from build123d import *

# Parameters (mm, degrees)
BOSS_EXTRUDE1_DEPTH      = 25
BOSS_EXTRUDE2_DEPTH      = 5
BOSS_EXTRUDE2_DEPTH_BACK = 40
SKETCH6_R                = 2
CUT_EXTRUDE2_DEPTH       = 56.302200077
SKETCH7_R                = 11.5
CUT_EXTRUDE3_DEPTH       = 59.434436194
CHAMFER3_SIZE            = 2
CHAMFER4_SIZE            = 8.660254038
CHAMFER4_SIZE_2          = 5
CUT_EXTRUDE4_DEPTH       = 0.5
CUT_EXTRUDE5_DEPTH       = 0.5


with BuildPart() as part:
    # Sketch1 → Boss-Extrude1 (new, symmetric)
    with BuildSketch(Plane.XY):
        Polygon((10.103629711, 17.5), (-10.103629711, 17.5), (-20.207259422, 0), (-10.103629711, -17.5), (10.103629711, -17.5), (20.207259422, 0), align=None)
    extrude(amount=BOSS_EXTRUDE1_DEPTH, both=True)

    # Sketch2 → Boss-Extrude2 (add, two sides: drawn at the far end of the back side and taken through both)
    with BuildSketch(Plane(origin=(0, 17.5, 0), x_dir=(1, 0, 0), z_dir=(0, 1, 0)).offset(-BOSS_EXTRUDE2_DEPTH_BACK)):
        with BuildLine():
            Line((-4.788486146, -5.353793539), (-4.788486146, 5.353793539))
            ThreePointArc((-4.788486146, 5.353793539), (0, 10.142279685), (4.788486146, 5.353793539))
            Line((4.788486146, 5.353793539), (4.788486146, -5.353793539))
            ThreePointArc((4.788486146, -5.353793539), (0, -10.142279685), (-4.788486146, -5.353793539))
        make_face()
    extrude(amount=BOSS_EXTRUDE2_DEPTH + BOSS_EXTRUDE2_DEPTH_BACK)

    # Sketch6 → Cut-Extrude2 (cut, through all)
    with BuildSketch(Plane(origin=(0, 22.5, 0), x_dir=(1, 0, 0), z_dir=(0, 1, 0))):
        with Locations(Location((0, -2.5, 0), (0, 0, 270))):
            Circle(SKETCH6_R)
        with Locations(Location((0, 2.5, 0), (0, 0, 270))):
            Circle(SKETCH6_R)
    extrude(amount=-CUT_EXTRUDE2_DEPTH, mode=Mode.SUBTRACT)

    # Sketch7 → Cut-Extrude3 (cut, through all)
    with BuildSketch(Plane(origin=(0, 0, -25), x_dir=(-1, 0, 0), z_dir=(0, 0, -1))):
        Circle(SKETCH7_R)
    extrude(amount=-CUT_EXTRUDE3_DEPTH, mode=Mode.SUBTRACT)

    # Chamfer3
    chamfer3_edges = [part.edges().sort_by_distance(p)[0] for p in [
        (-15.155444566, 8.75, 25),
        (-15.155444566, -8.75, 25),
        (0, -17.5, 25),
        (15.155444566, -8.75, 25),
        (15.155444566, 8.75, 25),
        (11.5, 0, 25),
        (11.5, 0, -25),
        (15.155444566, -8.75, -25),
        (0, -17.5, -25),
        (-15.155444566, -8.75, -25),
        (0, 17.5, 25),
        (-15.155444566, 8.75, -25),
        (0, 17.5, -25),
        (15.155444566, 8.75, -25),
    ]]
    chamfer(chamfer3_edges, length=CHAMFER3_SIZE)

    # Chamfer4
    # the kernel refuses this chamfer: 8.660254038, 5 mm, written as the material it adds along each edge
    with BuildSketch(Plane(origin=(4.788486146, -17.5, -5.353793539), x_dir=(0.9998132206222078, 0.019326765612700893, 0), z_dir=(0, 0, 1))) as chamfer4_piece_1_section:
        Polygon((CHAMFER4_SIZE * 0.999813220604, -CHAMFER4_SIZE * 0.0193267656124), (-CHAMFER4_SIZE_2 * 0.0193267656127, -CHAMFER4_SIZE_2 * 0.999813220622), (0, 0), align=None)
    chamfer4_piece_1 = extrude(amount=10.707587077, mode=Mode.PRIVATE)
    chamfer4_piece_1 = split(chamfer4_piece_1, bisect_by=Plane(origin=(8.460633685, -20.345752593, 0), z_dir=(-0.8660254037844387, 0.4999999999999999, 0)), keep=Keep.TOP, mode=Mode.PRIVATE)
    chamfer4_piece_1 = split(chamfer4_piece_1, bisect_by=Plane(origin=(6.722843937, -22.5, 0), z_dir=(0, 1, 0)), keep=Keep.TOP, mode=Mode.PRIVATE)
    add(chamfer4_piece_1)
    with BuildSketch(Plane(origin=(0, -17.5, -5.353793539), x_dir=(-1, 0, 0), z_dir=(0, 0, 1))) as chamfer4_piece_2_section:
        Polygon((4.788486146 + CHAMFER4_SIZE, 0), (4.788486146, CHAMFER4_SIZE_2), (4.788486146, 0), align=None)
    chamfer4_piece_2 = revolve(axis=Axis((0, -17.5, -5.353793539), (0, -1, 0)), revolution_arc=180, mode=Mode.PRIVATE)
    chamfer4_piece_2 = split(chamfer4_piece_2, bisect_by=Plane(origin=(6.935994124, -22.986505777, -10.917233829), z_dir=(-0.8660254037844387, 0.4999999999999999, 0)), keep=Keep.TOP, mode=Mode.PRIVATE)
    chamfer4_piece_2 = split(chamfer4_piece_2, bisect_by=Plane(origin=(-6.935994098, -22.986505822, -10.917233829), z_dir=(0.8660254037844385, 0.5000000000000003, 0)), keep=Keep.TOP, mode=Mode.PRIVATE)
    chamfer4_piece_2 = split(chamfer4_piece_2, bisect_by=Plane(origin=(5.2e-08, -22.5, -10.917233829), z_dir=(0, 1, 0)), keep=Keep.TOP, mode=Mode.PRIVATE)
    add(chamfer4_piece_2)
    with BuildSketch(Plane(origin=(0, -17.5, 5.353793539), x_dir=(1, 0, 0), z_dir=(0, 0, -1))) as chamfer4_piece_3_section:
        Polygon((4.788486146 + CHAMFER4_SIZE, 0), (4.788486146, CHAMFER4_SIZE_2), (4.788486146, 0), align=None)
    chamfer4_piece_3 = revolve(axis=Axis((0, -17.5, 5.353793539), (0, -1, 0)), revolution_arc=180, mode=Mode.PRIVATE)
    chamfer4_piece_3 = split(chamfer4_piece_3, bisect_by=Plane(origin=(6.935994128, -22.98650577, 10.917233836), z_dir=(-0.8660254037844387, 0.4999999999999999, 0)), keep=Keep.TOP, mode=Mode.PRIVATE)
    chamfer4_piece_3 = split(chamfer4_piece_3, bisect_by=Plane(origin=(-6.935994097, -22.986505824, 10.917233836), z_dir=(0.8660254037844385, 0.5000000000000003, 0)), keep=Keep.TOP, mode=Mode.PRIVATE)
    chamfer4_piece_3 = split(chamfer4_piece_3, bisect_by=Plane(origin=(6.2e-08, -22.5, 10.917233836), z_dir=(0, 1, 0)), keep=Keep.TOP, mode=Mode.PRIVATE)
    add(chamfer4_piece_3)
    with BuildSketch(Plane(origin=(-4.788486146, -17.5, 5.353793539), x_dir=(-0.999813220622208, 0.019326765612700497, 0), z_dir=(0, 0, -1))) as chamfer4_piece_4_section:
        Polygon((CHAMFER4_SIZE * 0.999813220604, -CHAMFER4_SIZE * 0.0193267656124), (-CHAMFER4_SIZE_2 * 0.0193267656127, -CHAMFER4_SIZE_2 * 0.999813220622), (0, 0), align=None)
    chamfer4_piece_4 = extrude(amount=10.707587077, mode=Mode.PRIVATE)
    chamfer4_piece_4 = split(chamfer4_piece_4, bisect_by=Plane(origin=(-8.460633685, -20.345752593, 0), z_dir=(0.8660254037844385, 0.5000000000000003, 0)), keep=Keep.TOP, mode=Mode.PRIVATE)
    chamfer4_piece_4 = split(chamfer4_piece_4, bisect_by=Plane(origin=(-6.722843937, -22.5, 0), z_dir=(0, 1, 0)), keep=Keep.TOP, mode=Mode.PRIVATE)
    add(chamfer4_piece_4)
    with BuildSketch(Plane(origin=(-4.788486146, 17.5, -5.353793539), x_dir=(-0.999813220622208, -0.019326765612700497, 0), z_dir=(0, 0, 1))) as chamfer4_piece_5_section:
        Polygon((CHAMFER4_SIZE * 0.999813220604, -CHAMFER4_SIZE * 0.0193267656124), (-CHAMFER4_SIZE_2 * 0.0193267656127, -CHAMFER4_SIZE_2 * 0.999813220622), (0, 0), align=None)
    chamfer4_piece_5 = extrude(amount=10.707587077, mode=Mode.PRIVATE)
    chamfer4_piece_5 = split(chamfer4_piece_5, bisect_by=Plane(origin=(-8.460633685, 20.345752593, 0), z_dir=(0.8660254037844388, -0.49999999999999983, 0)), keep=Keep.TOP, mode=Mode.PRIVATE)
    chamfer4_piece_5 = split(chamfer4_piece_5, bisect_by=Plane(origin=(-6.722843937, 22.5, 0), z_dir=(0, -1, 0)), keep=Keep.TOP, mode=Mode.PRIVATE)
    add(chamfer4_piece_5)
    with BuildSketch(Plane(origin=(0, 17.5, 5.353793539), x_dir=(1, 0, 0), z_dir=(0, 0, -1))) as chamfer4_piece_6_section:
        Polygon((4.788486146 + CHAMFER4_SIZE, 0), (4.788486146, -CHAMFER4_SIZE_2), (4.788486146, 0), align=None)
    chamfer4_piece_6 = revolve(axis=Axis((0, 17.5, 5.353793539), (0, -1, 0)), revolution_arc=180, mode=Mode.PRIVATE)
    chamfer4_piece_6 = split(chamfer4_piece_6, bisect_by=Plane(origin=(6.935994103, 22.986505812, 10.917233841), z_dir=(-0.8660254037844387, -0.5000000000000003, 0)), keep=Keep.TOP, mode=Mode.PRIVATE)
    chamfer4_piece_6 = split(chamfer4_piece_6, bisect_by=Plane(origin=(-6.935994125, 22.986505774, 10.917233841), z_dir=(0.8660254037844388, -0.49999999999999983, 0)), keep=Keep.TOP, mode=Mode.PRIVATE)
    chamfer4_piece_6 = split(chamfer4_piece_6, bisect_by=Plane(origin=(-4.4e-08, 22.5, 10.917233841), z_dir=(0, -1, 0)), keep=Keep.TOP, mode=Mode.PRIVATE)
    add(chamfer4_piece_6)
    with BuildSketch(Plane(origin=(0, 17.5, -5.353793539), x_dir=(-1, 0, 0), z_dir=(0, 0, 1))) as chamfer4_piece_7_section:
        Polygon((4.788486146 + CHAMFER4_SIZE, 0), (4.788486146, -CHAMFER4_SIZE_2), (4.788486146, 0), align=None)
    chamfer4_piece_7 = revolve(axis=Axis((0, 17.5, -5.353793539), (0, -1, 0)), revolution_arc=180, mode=Mode.PRIVATE)
    chamfer4_piece_7 = split(chamfer4_piece_7, bisect_by=Plane(origin=(6.935994097, 22.986505823, -10.917233827), z_dir=(-0.8660254037844387, -0.5000000000000003, 0)), keep=Keep.TOP, mode=Mode.PRIVATE)
    chamfer4_piece_7 = split(chamfer4_piece_7, bisect_by=Plane(origin=(-6.93599412, 22.986505784, -10.917233827), z_dir=(0.8660254037844388, -0.49999999999999983, 0)), keep=Keep.TOP, mode=Mode.PRIVATE)
    chamfer4_piece_7 = split(chamfer4_piece_7, bisect_by=Plane(origin=(-4.6e-08, 22.5, -10.917233827), z_dir=(0, -1, 0)), keep=Keep.TOP, mode=Mode.PRIVATE)
    add(chamfer4_piece_7)
    with BuildSketch(Plane(origin=(4.788486146, 17.5, 5.353793539), x_dir=(0.999813220622208, -0.019326765612700497, 0), z_dir=(0, 0, -1))) as chamfer4_piece_8_section:
        Polygon((CHAMFER4_SIZE * 0.999813220604, -CHAMFER4_SIZE * 0.0193267656124), (-CHAMFER4_SIZE_2 * 0.0193267656127, -CHAMFER4_SIZE_2 * 0.999813220622), (0, 0), align=None)
    chamfer4_piece_8 = extrude(amount=10.707587077, mode=Mode.PRIVATE)
    chamfer4_piece_8 = split(chamfer4_piece_8, bisect_by=Plane(origin=(8.460633685, 20.345752593, 0), z_dir=(-0.8660254037844387, -0.5000000000000003, 0)), keep=Keep.TOP, mode=Mode.PRIVATE)
    chamfer4_piece_8 = split(chamfer4_piece_8, bisect_by=Plane(origin=(6.722843937, 22.5, 0), z_dir=(0, -1, 0)), keep=Keep.TOP, mode=Mode.PRIVATE)
    add(chamfer4_piece_8)

    # Sketch8 → Cut-Extrude4 (cut)
    with BuildSketch(Plane(origin=(15.155444566, -8.75, 0), x_dir=(0, 0, -1), z_dir=(0.8660254037844387, -0.49999999999999983, 0))):
        Polygon((4.862923627, 0.810905121), (4.862923627, 1.689163545), (7.714387746, -0.02362609), (4.862923627, -1.736415726), (4.862923627, -0.858157301), (-7.055157189, -0.858157301), (-7.055157189, 0.810905121), align=None)
    extrude(amount=-CUT_EXTRUDE4_DEPTH, mode=Mode.SUBTRACT)

    # Sketch9 → Cut-Extrude5 (cut)
    with BuildSketch(Plane(origin=(-15.155444566, 8.75, 0), x_dir=(0, 0, 1), z_dir=(-0.8660254037844389, 0.49999999999999983, 0))):
        Polygon((-4.515922363, -0.834531211), (-4.515922363, -1.712789635), (-7.367386481, 0), (-4.515922363, 1.712789635), (-4.515922363, 0.834531211), (7.402158453, 0.834531211), (7.402158453, -0.834531211), align=None)
    extrude(amount=-CUT_EXTRUDE5_DEPTH, mode=Mode.SUBTRACT)


solid = part.part
Build history of the part. All positions in model axes, mm. Round coordinates to 2 decimals unless told otherwise and drop trailing zeros. Loops run counter-clockwise (first coordinate to the right, second up) from the corner with the lowest first, then second, coordinate; pieces in that order, holes last. Notation, with made-up numbers: (23, 46) -> (63, 46) arc R21 ccw to (63, 55) -> close; hole circle Ø7 at (-4.5, 89). An arc over 180 degrees is marked (long way). Answer in a Markdown table with one row per item.
Item 1: Drill centre lines: L1, parallel to Z at x = 0, y = 15; L2, parallel to Z at x = 0.5, y = 18.5; L3, parallel to Y at x = 3, z = -17.5. Where is each one in solid material? Low to high. Write a range as [from, to].
Answers below:
| item | result |
|---|---|
| L1 | z = [-25, -4.5], [-0.5, 0.5], [4.5, 25] |
| L2 | z = [-17.06, -4.44], [-0.56, 0.56], [4.44, 17.06] |
| L3 | y = [-18.04, -11.1], [11.1, 18.04] |
Item 2: Pin check, flat tips, straight feed: pin 1 (2.5 mm diameter, centred on x = -2.5, z = 19, fed in from -Y); pin 2 (3 mm diameter, centred on x = 0, z = 2.5, fed in from +Y); pin 3 (3 mm diameter, centred on x = 7, z = -3, fed in from -Y); pin 4 (1 mm diameter, centred on x = 12, z = 10, fed in from +Y). Stop position of each tip, or through.
Answers below:
| item | result |
|---|---|
| pin 1 | stops at y = -17.98 |
| pin 2 | passes through |
| pin 3 | stops at y = -22.09 |
| pin 4 | stops at y = 15.08 |
Item 3: Saw through at B-B (x = 0). State how many separate pieces and enclosed holes the cut face has, and give its area (3 significant figures).
Answers below:
| item | result |
|---|---|
| separate pieces | 6 |
| enclosed holes | 0 |
| area | 697 mm² |
Item 4: Mould opens along Y. For faces 1 (the flat face through (14.51, -9.38, -6.31)), 2 (the flat face through (-0.1, -16.5, -24)), 3 (the flat face through (14.37, 8.13, -23.99)), 4 (the flat face through (14.723, -8.5, -0.433)) say: +Y half, -Y half, draft (parallel to the pull), parting line (faces both ways), or undercut.
Answers below:
| item | result |
|---|---|
| face 1 | undercut |
| face 2 | -Y half |
| face 3 | +Y half |
| face 4 | undercut |
Item 5: Saw through at C-C (y = -16.5). Write the cut outline in (x, z), and give its area (3 significant figures).
Answers below:
| item | result |
|---|---|
| outline | (-10.68, -23) -> (-9.53, -24) -> (9.53, -24) -> (10.68, -23) -> (10.68, 23) -> (9.53, 24) -> (-9.53, 24) -> (-10.68, 23) -> close; hole circle Ø4 at (0, -2.5); hole circle Ø4 at (0, 2.5) |
| area | 998 mm² |
Item 6: Saw through at A-A (z = 2.5). Write the cut outline in (x, y).
Answers below:
| item | result |
|---|---|
| outline | (-20.21, 0) -> (-8.43, -20.4) -> (-4.79, -22.5) -> (-2, -22.5) -> (-2, -11.32) arc R11.5 cw to (-2, 11.32) -> (-2, 22.5) -> (-4.79, 22.5) -> (-8.43, 20.4) -> (-14.74, 9.47) -> (-14.31, 9.22) -> (-15.14, 7.78) -> (-15.57, 8.03) -> close; (2, -22.5) -> (4.79, -22.5) -> (8.43, -20.4) -> (14.73, -9.49) -> (14.29, -9.24) -> (15.13, -7.8) -> (15.56, -8.05) -> (20.21, 0) -> (8.43, 20.4) -> (4.79, 22.5) -> (2, 22.5) -> (2, 11.32) arc R11.5 cw to (2, -11.32) -> close |
